Geometry: final body of the model. Coordinates: model frame, mm. Give positions to 0.01 mm unless a question says otherwise; leave off trailing zeros. Order: outer loops, then holes, each group sorted by start corner. A loop starts at its lowest first (then second) coordinate and runs counter-clockwise, first axis right, second up. Notation, with made-up numbers: (64.5, 13.5) -> (103.5, 13.5) arc R10 cw to (103.5, 23.5) -> close; hole circle Ø3 at (67.5, -2.75). An arc over 180 degrees is marked (long way). Answer in a Markdown table with one row per item. Add a question column.
Q1. Line query: line 1 along Z through (x, y) = (0, 1.6); line 2 along Z through (x, y) = (-1.3, 1.1). Output: solid intervals per line, ascending. Write a range as from..to.
Q2. Cut plane B-B on x = 0. Return the cut outline in (y, z).
Q3. Pull-direction query (X, two-part tool) for faces 1 (the face through (-1.431, 1.545, 0.593)), 2 (the face through (0.33, 1.75, -2.52)), 3 (the face through (0.251, 1.503, -1.914)); classes: +X half, -X half, draft (parallel to the pull), parting line (faces both ways), or undercut.
Q4. Cut plane A-A on y = 0.3. Return the cut outline in (x, z), and give its area (3 significant figures).
Q5. Contact query for flat-ended pins moving along their axis: P1, Ø3, axis at x = 0, z = 0, coming from the +Y side; P2, Ø1, axis at x = 1, y = 1, coming from the +Z side; P3, Ø1, axis at x = -1, y = 2.5, coming from the -Z side. Output: stop coordinate, or through.
Q6. Cut plane C-C on z = 0. Return the cut outline in (x, y).
from build123d import *


with BuildPart() as part:
    # Sketch1 → Revolve1 (revolve)
    with BuildSketch(Plane.XY):
        with BuildLine():
            Line((-1.5494, 0), (-1.5494, 3.048))
            Line((-1.5494, 3.048), (0, 3.048))
            Line((0, 3.048), (0, 3.81))
            ThreePointArc((0, 3.81), (-1.058992944, 3.841119954), (-2.114331034, 3.934372414))
            ThreePointArc((-2.114331034, 3.934372414), (-2.412122623, 3.84076295), (-2.54, 3.556))
            Line((-2.54, 3.556), (-2.54, 0))
            Line((-2.54, 0), (-2.159, 0))
            Line((-2.159, 0), (-2.159, 3.048))
            Line((-2.159, 3.048), (-1.9304, 3.048))
            Line((-1.9304, 3.048), (-1.9304, 0))
            Line((-1.9304, 0), (-1.5494, 0))
        make_face()
    revolve(axis=Axis((0, 0, 0), (0, -1, 0)))


solid = part.part
Completed:
| question | item | result |
|---|---|---|
| 1 | line 1 | z = -2.54..-2.16, -1.93..-1.55, 1.55..1.93, 2.16..2.54 |
| 1 | line 2 | z = -2.18..-1.72, -1.43..-0.84, 0.84..1.43, 1.72..2.18 |
| 2 | outline | (0, -2.54) -> (3.56, -2.54) arc R0.38 ccw to (3.93, -2.11) arc R18.03 cw to (3.93, 2.11) arc R0.38 ccw to (3.56, 2.54) -> (0, 2.54) -> (0, 2.16) -> (3.05, 2.16) -> (3.05, 1.93) -> (0, 1.93) -> (0, 1.55) -> (3.05, 1.55) -> (3.05, -1.55) -> (0, -1.55) -> (0, -1.93) -> (3.05, -1.93) -> (3.05, -2.16) -> (0, -2.16) -> close |
| 3 | face 1 | undercut |
| 3 | face 2 | parting line |
| 3 | face 3 | undercut |
| 4 | outline | circle Ø5.08 at (0, 0); circle Ø3.86 at (0, 0); hole circle Ø4.32 at (0, 0); hole circle Ø3.1 at (0, 0) |
| 4 | area | 9.79 mm² |
| 5 | P1 | stops at y = 3.87 |
| 5 | P2 | stops at z = 2.49 |
| 5 | P3 | stops at z = -2.49 |
| 6 | outline | (-2.54, 0) -> (-2.16, 0) -> (-2.16, 3.05) -> (-1.93, 3.05) -> (-1.93, 0) -> (-1.55, 0) -> (-1.55, 3.05) -> (1.55, 3.05) -> (1.55, 0) -> (1.93, 0) -> (1.93, 3.05) -> (2.16, 3.05) -> (2.16, 0) -> (2.54, 0) -> (2.54, 3.56) arc R0.38 ccw to (2.11, 3.93) arc R18.03 cw to (-2.11, 3.93) arc R0.38 ccw to (-2.54, 3.56) -> close |
